Read the model definition and answer for the solid it produces. Units are mm, in the model's axes. Face numbers are marked on the shaded views. A direction names the side the tool comes from. Coordinates: 2 decimals unless noted, no trailing zeros. Write each loop counter-clockwise with the first axis right and the second up, starting at its lowest first coordinate (ties: lowest second). Pieces come first, ordered by that corner, then holes.
Item 1: Section C-C (y = 1.3) is taken. Give the vertices of the cut face in (x, z), then the cut area to 3 significant figures.
Item 2: Section D-D (y = -1.1) is taken. Give the vertices of the cut face in (x, z).
Item 3: Straight lines are drawn through the part: probe 1 along Y at (x, z) = (3.5, -2.25); probe 2 along Y at (x, z) = (6.25, -0.75); probe 3 along Z at (x, y) = (3, -1.8). For each, find the intervals that lie inside material, in ascending order.
Item 4: Determine the mould class of the marked faces 1, 2, 3 and 4 for opening direction Z: released by +Z, released by -Z, zero draft, split by the parting line, or undercut.
Item 5: A tool of negligible diameter and unlimited length cuts with its end or side. For the marked faces 5 and 6, from which of +Z, -Z, +X, -X, +Y, -Y can it reach the whole face along a straight path? Write none if from no direction.
Item 6: Section B-B (x = 1.25) is taken. Give the vertices of the cut face in (y, z).
Item 7: Each of these flat-tipped pins is pushed along its axis until it touches: P1, Ø3, axis at x = 1.5, z = -4.5, coming from the -Y side; P2, Ø1.5, axis at y = 0.5, z = -5, coming from the +X side; P3, Ø1.5, axis at y = 1, z = -6.5, coming from the -X side; P4, Ø1, axis at x = 4, y = -1.5, coming from the +Z side. Where does it stop, or does it pass through?
Item 8: Section A-A (y = 0.1) is taken. Give the vertices of the cut face in (x, z), then the cut area to 3 significant figures.
from build123d import *

# Parameters (mm, degrees)
SKETCH1_W               = 8
SKETCH1_H               = 8
BOSS_EXTRUDE1_DEPTH     = 3
CUT_EXTRUDE1_DEPTH      = 12.704699911
CUT_EXTRUDE1_DEPTH_BACK = 12.704699911
CUT_EXTRUDE2_DEPTH      = 11
SKETCH4_R               = 1.75
CUT_EXTRUDE3_DEPTH      = 0.4
SKETCH5_W               = 8
SKETCH5_H               = 1
BOSS_EXTRUDE2_DEPTH     = 2
FILLET1_R               = 4
CUT_EXTRUDE4_DEPTH      = 0.4
CUT_EXTRUDE5_DEPTH      = 0.4


with BuildPart() as part:
    # Sketch1 → Boss-Extrude1 (new body)
    with BuildSketch(Plane(origin=(0, 0, 0), x_dir=(1, 0, 0), z_dir=(0, 1, 0))):
        with Locations((4, 4)):
            Rectangle(SKETCH1_W, SKETCH1_H)
    extrude(amount=BOSS_EXTRUDE1_DEPTH)

    # Sketch2 → Cut-Extrude1 (cut, two sides: drawn at the far end of the back side and taken through both)
    with BuildSketch(Plane.XY.offset(-CUT_EXTRUDE1_DEPTH_BACK)):
        Polygon((0, 0), (0.6, 3), (0, 3), align=None)
        Polygon((8, 0), (7.4, 3), (8, 3), align=None)
    extrude(amount=CUT_EXTRUDE1_DEPTH + CUT_EXTRUDE1_DEPTH_BACK, mode=Mode.SUBTRACT)

    # Sketch3 → Cut-Extrude2 (cut)
    with BuildSketch(Plane(origin=(0, 0, 0), x_dir=(0, 0, -1), z_dir=(1, 0, 0))):
        Polygon((0, 0), (0.6, 3), (0, 3), align=None)
        Polygon((8, 3), (7.4, 3), (8, 0), align=None)
    extrude(amount=CUT_EXTRUDE2_DEPTH, mode=Mode.SUBTRACT)

    # Sketch4 → Cut-Extrude3 (cut)
    with BuildSketch(Plane.XZ):
        with Locations(Location((4, -3.75, 0), (0, 0, 270))):
            Circle(SKETCH4_R)
    extrude(amount=-CUT_EXTRUDE3_DEPTH, mode=Mode.SUBTRACT)

    # Sketch5 → Boss-Extrude2 (add)
    with BuildSketch(Plane.XZ):
        with Locations((4, -7.5)):
            Rectangle(SKETCH5_W, SKETCH5_H)
    extrude(amount=BOSS_EXTRUDE2_DEPTH)

    # Fillet1
    # the kernel refuses this fillet: 4 mm, written as the material it takes off along each edge
    with BuildSketch(Plane(origin=(8, -2, -16.660254038), x_dir=(0, 1, 0), z_dir=(0, 0, 1)), Plane(origin=(0, -2, 1.660254038), x_dir=(0, 1, 0), z_dir=(0, 0, -1))) as fillet1_piece_1:
        with BuildLine():
            CenterArc((4, 3.464101615), FILLET1_R, 180, 60)
            Line((0, 3.464101615), (-0.08, 3.464101615))
            Line((-0.08, 3.464101615), (-0.08, 0))
            Line((-0.08, 0), (0, -0.08))
            ThreePointArc((0, -0.08), (1, -0.08), (1.96, -0.069282032))
            Line((1.96, -0.069282032), (2, 0))
        make_face()
    extrude(amount=18.320508076, mode=Mode.SUBTRACT)

    # Sketch6 → Cut-Extrude4 (cut)
    with BuildSketch(Plane(origin=(0, 3, 0), x_dir=(1, 0, 0), z_dir=(0, 1, 0))):
        with BuildLine():
            Line((4.053794593, 3.505457585), (4.053794593, 4.172124252))
            Line((4.053794593, 4.172124252), (5.797384337, 4.172124252))
            Line((5.797384337, 4.172124252), (5.797384337, 2.564752457))
            add(Edge.make_bspline(
                [(5.797384337, 2.564752457), (5.775440275, 2.544992361), (5.730582172, 2.504598726), (5.657391115, 2.447633596), (5.576814656, 2.393249062), (5.489339896, 2.340343698), (5.394785806, 2.289343315), (5.293529517, 2.239537607), (5.185384208, 2.19141366), (5.032450931, 2.131128575), (4.835594452, 2.065533422), (4.594933471, 2.008496304), (4.352368706, 1.973513189), (4.190125473, 1.969167013), (4.109083055, 1.966996047)],
                knots=[0, 0, 0, 0, 0.581799769, 1.189316438, 1.825828404, 2.496525428, 3.203088405, 3.942228803, 4.719818701, 5.534979611, 7.181138583, 8.803804008, 10.403462225, 12, 12, 12, 12], degree=3))
            add(Edge.make_bspline(
                [(4.109083055, 1.966996047), (4.058312627, 1.967758979), (3.958229013, 1.969262944), (3.810482794, 1.981368296), (3.667847904, 2.002080495), (3.530208107, 2.031409962), (3.397097502, 2.066765974), (3.26907094, 2.111868039), (3.146582956, 2.166009466), (3.028523806, 2.226338905), (2.917094396, 2.295632176), (2.812187083, 2.371432832), (2.714561168, 2.454400196), (2.624566637, 2.544701507), (2.540998329, 2.641714843), (2.464831298, 2.745902822), (2.396526155, 2.857385727), (2.335239765, 2.974765127), (2.280716867, 3.097008702), (2.234709094, 3.223154334), (2.194374003, 3.351370526), (2.161222966, 3.482107416), (2.136875151, 3.615790052), (2.117947657, 3.751799892), (2.107781758, 3.890986734), (2.105984472, 3.984609884), (2.105076645, 4.031899893)],
                knots=[0, 0, 0, 0, 1.124918047, 2.217548049, 3.282233239, 4.316494221, 5.334437038, 6.332151046, 7.320712088, 8.300141923, 9.267552434, 10.225301062, 11.165776911, 12.103230934, 13.047553934, 14.000517593, 14.959782875, 15.941944936, 16.932894943, 17.923491392, 18.915624898, 19.910402922, 20.909870877, 21.92519501, 22.95199481, 24, 24, 24, 24], degree=3))
            add(Edge.make_bspline(
                [(2.105076645, 4.031899893), (2.105812881, 4.082940857), (2.107264322, 4.183564655), (2.119773705, 4.33228546), (2.139199297, 4.476648194), (2.168656936, 4.616390773), (2.20449512, 4.75216369), (2.248233589, 4.883877531), (2.301822866, 5.010556427), (2.361436063, 5.133283761), (2.429297714, 5.250362339), (2.505977563, 5.360290437), (2.589206445, 5.464176802), (2.680629029, 5.560371285), (2.779923369, 5.648827012), (2.886080088, 5.730522243), (2.998844963, 5.806865303), (3.079553832, 5.849911113), (3.120301004, 5.871643482)],
                knots=[0, 0, 0, 0, 1.105010302, 2.178452875, 3.229459892, 4.257086284, 5.268538906, 6.268935615, 7.259234261, 8.24469117, 9.221745683, 10.185929258, 11.144249683, 12.101504986, 13.055838221, 14.020611351, 15.000673771, 16, 16, 16, 16], degree=3))
            add(Edge.make_bspline(
                [(3.120301004, 5.871643482), (3.152638085, 5.887700047), (3.218317351, 5.920312247), (3.322813337, 5.959248923), (3.432101667, 5.994677516), (3.547832356, 6.021111591), (3.6692195, 6.042829226), (3.796209305, 6.059036287), (3.929210312, 6.067547239), (4.019595582, 6.068879104), (4.065813824, 6.069560149)],
                knots=[0, 0, 0, 0, 0.887969848, 1.803539625, 2.741143579, 3.713741423, 4.722068772, 5.775476617, 6.8624965, 8, 8, 8, 8], degree=3))
            add(Edge.make_bspline(
                [(4.065813824, 6.069560149), (4.125403824, 6.06867255), (4.241295356, 6.066946335), (4.410256532, 6.05256252), (4.569271079, 6.027772487), (4.718560435, 5.993629866), (4.857802985, 5.949731518), (4.986759025, 5.895763799), (5.106220057, 5.832812796), (5.214455834, 5.758355608), (5.313666102, 5.676257846), (5.403591975, 5.586419647), (5.48426965, 5.488707943), (5.555752499, 5.383614392), (5.617477906, 5.2707046), (5.670549966, 5.151008328), (5.714234697, 5.023616882), (5.73534656, 4.935145779), (5.746102286, 4.89007297)],
                knots=[0, 0, 0, 0, 1.271135529, 2.472123572, 3.614091059, 4.701890498, 5.736279567, 6.724681829, 7.680621489, 8.611506429, 9.52200816, 10.424540711, 11.318996785, 12.221421405, 13.131851814, 14.060431888, 15.011860567, 16, 16, 16, 16], degree=3))
            Line((5.746102286, 4.89007297), (4.976871517, 4.736226816))
            add(Edge.make_bspline(
                [(4.976871517, 4.736226816), (4.969254672, 4.761468809), (4.95422678, 4.81127079), (4.925094227, 4.882758251), (4.891539922, 4.949961192), (4.853483379, 5.013366036), (4.810541206, 5.072582433), (4.761675926, 5.126971617), (4.709961453, 5.179014495), (4.652020351, 5.225088646), (4.590259767, 5.266624284), (4.52537561, 5.304078684), (4.455901775, 5.334453158), (4.382811411, 5.358892727), (4.306461756, 5.37964837), (4.225856415, 5.392413169), (4.141900573, 5.402040295), (4.084540473, 5.402606041), (4.055397158, 5.402893482)],
                knots=[0, 0, 0, 0, 1.027736275, 2.027704492, 3.005900071, 3.954421694, 4.908588141, 5.853155543, 6.803277083, 7.766271258, 8.734041521, 9.704274878, 10.683578894, 11.68490234, 12.708089448, 13.76461009, 14.864251086, 16, 16, 16, 16], degree=3))
            add(Edge.make_bspline(
                [(4.055397158, 5.402893482), (4.01128773, 5.401716629), (3.925204424, 5.399419898), (3.799534269, 5.384433236), (3.680976007, 5.357770589), (3.569219615, 5.320994553), (3.46406021, 5.273789934), (3.366918824, 5.2143961), (3.275376693, 5.146327474), (3.192038786, 5.066438045), (3.116460773, 4.976859168), (3.051034483, 4.876522357), (2.996567377, 4.765751945), (2.951955713, 4.645104141), (2.91643531, 4.514573915), (2.892338718, 4.373699188), (2.876594443, 4.222696077), (2.875085403, 4.118480819), (2.874307414, 4.064752457)],
                knots=[0, 0, 0, 0, 1.043810997, 2.037086103, 2.989314757, 3.91471467, 4.817033861, 5.710208705, 6.603920097, 7.511448416, 8.435617211, 9.371747005, 10.338444094, 11.350425613, 12.411431869, 13.5347293, 14.729025275, 16, 16, 16, 16], degree=3))
            add(Edge.make_bspline(
                [(2.874307414, 4.064752457), (2.875118698, 4.00702506), (2.876695474, 3.894828493), (2.892027057, 3.732262921), (2.917247643, 3.580803592), (2.95342224, 3.44064155), (2.998941149, 3.311279521), (3.053656914, 3.192304252), (3.121182779, 3.085923464), (3.197244894, 2.990004781), (3.28225913, 2.906191636), (3.37384152, 2.833121051), (3.471482188, 2.77119638), (3.576081527, 2.721395085), (3.686320303, 2.681751972), (3.80321198, 2.653959398), (3.926408504, 2.636695674), (4.010734238, 2.634687946), (4.053794593, 2.633662713)],
                knots=[0, 0, 0, 0, 1.318042826, 2.561693173, 3.724929596, 4.821196409, 5.862977565, 6.853497791, 7.804600806, 8.73339865, 9.643480846, 10.524649628, 11.404635349, 12.277659519, 13.165160235, 14.075017549, 15.017020959, 16, 16, 16, 16], degree=3))
            add(Edge.make_bspline(
                [(4.053794593, 2.633662713), (4.097408334, 2.634875039), (4.185053042, 2.637311287), (4.316328539, 2.657956024), (4.448117665, 2.68833542), (4.577327471, 2.734163302), (4.70281192, 2.786727561), (4.819965055, 2.847306941), (4.929675356, 2.910453005), (4.995733738, 2.959668979), (5.028153568, 2.98382297)],
                knots=[0, 0, 0, 0, 0.993821502, 1.997150276, 3.023717651, 4.073291794, 5.118404464, 6.123376694, 7.078999408, 8, 8, 8, 8], degree=3))
            Line((5.028153568, 2.98382297), (5.028153568, 3.505457585))
            Line((5.028153568, 3.505457585), (4.053794593, 3.505457585))
        make_face()
    extrude(amount=-CUT_EXTRUDE4_DEPTH, mode=Mode.SUBTRACT)

    # Sketch7 → Cut-Extrude5 (cut)
    with BuildSketch(Plane(origin=(0, 3, 0), x_dir=(1, 0, 0), z_dir=(0, 1, 0))):
        Polygon((7.051946272, 3.224540865), (7.051946272, 0.93992548), (6.405792426, 0.93992548), (6.405792426, 1.23992548), (6.705792426, 1.23992548), (6.705792426, 2.924540865), (6.405792426, 2.924540865), (6.405792426, 3.224540865), align=None)
    extrude(amount=-CUT_EXTRUDE5_DEPTH, mode=Mode.SUBTRACT)


solid = part.part
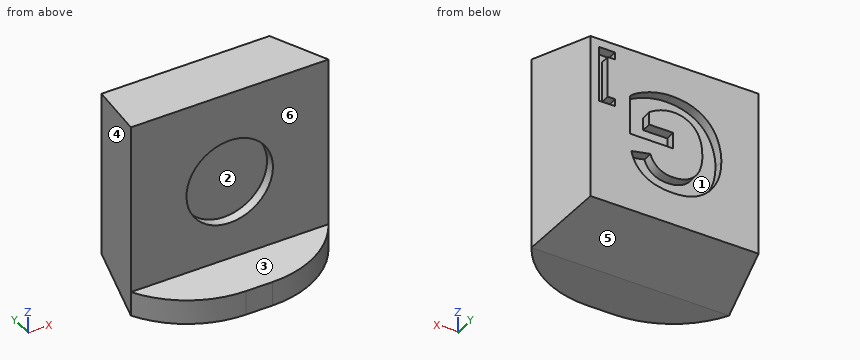
Established:
1. outline: (0.26, -7.74) - (7.74, -7.74) - (7.74, -0.26) - (0.26, -0.26) - close
1. area: 56.0 mm2
2. outline: (0.94, -8) - (7.06, -8) - (7.06, -7) - (0.94, -7) - close
3. probe 1: y = 0.4 to 2.6
3. probe 2: y = 0 to 3
3. probe 3: z = -8 to -7
4. face 1: undercut
4. face 2: undercut
4. face 3: released by +Z
4. face 4: zero draft
5. face 5: -Z, +X, -X, +Y
5. face 6: +Z, +X, -X, -Y
6. outline: (-1.33, -8) - (0, -8) - (3, -7.4) - (3, -0.6) - (0, 0) - (0, -7) - (-1.33, -7) - close
7. P1: stops at y = 0
7. P2: stops at x = 8
7. P3: stops at x = 0.05
7. P4: stops at z = -7
8. outline: (0.02, -7.98) - (7.98, -7.98) - (7.98, -0.02) - (0.02, -0.02) - close; hole circle Ø3.5 at (4, -3.75)
8. area: 53.7 mm2
